```python
from build123d import *

# Parameters (mm, degrees)
ESBO_O1_W                = 50
ESBO_O1_H                = 11
RESSALTO_EXTRUS_O1_DEPTH = 22.5
ESBO_O2_W                = 46
ESBO_O2_H                = 7
CORTE_EXTRUS_O1_DEPTH    = 20.5
ESBO_O3_W                = 10.97916057
ESBO_O3_H                = 2
CORTE_EXTRUS_O2_DEPTH    = 4
CORTE_EXTRUS_O3_DEPTH    = 4
ESBO_O9_W                = 50
ESBO_O9_H                = 4
RESSALTO_EXTRUS_O4_DEPTH = 7
ESBO_O13_R               = 1.5
CORTE_EXTRUS_O4_DEPTH    = 7
ESBO_O19_W               = 9
ESBO_O19_H               = 4
RESSALTO_EXTRUS_O5_DEPTH = 22.5


with BuildPart() as part:
    # Esboço1 → Ressalto-extrusão1 (new body)
    with BuildSketch(Plane(origin=(0, 0, 0), x_dir=(1, 0, 0), z_dir=(0, 1, 0))):
        Rectangle(ESBO_O1_W, ESBO_O1_H)
    extrude(amount=RESSALTO_EXTRUS_O1_DEPTH)

    # Esboço2 → Corte-extrusão1 (cut)
    with BuildSketch(Plane(origin=(0, 22.5, 0), x_dir=(1, 0, 0), z_dir=(0, 1, 0))):
        Rectangle(ESBO_O2_W, ESBO_O2_H)
    extrude(amount=-CORTE_EXTRUS_O1_DEPTH, mode=Mode.SUBTRACT)

    # Esboço3 → Corte-extrusão2 (cut)
    with BuildSketch(Plane(origin=(0, 22.5, 0), x_dir=(1, 0, 0), z_dir=(0, 1, 0))):
        with Locations((0, 4.5)):
            Rectangle(ESBO_O3_W, ESBO_O3_H)
    extrude(amount=-CORTE_EXTRUS_O2_DEPTH, mode=Mode.SUBTRACT)

    # Esboço5 → Corte-extrusão3 (cut)
    with BuildSketch(Plane.XY.offset(5.5)):
        with BuildLine():
            Line((-21, 22.5), (-4.5, 22.5))
            Line((-4.5, 22.5), (-4.5, 11.75))
            ThreePointArc((-4.5, 11.75), (-12.75, 3.5), (-21, 11.75))
            Line((-21, 11.75), (-21, 22.5))
        make_face()
        with BuildLine():
            Line((4.5, 22.5), (21, 22.5))
            Line((21, 22.5), (21, 11.75))
            ThreePointArc((21, 11.75), (12.75, 3.5), (4.5, 11.75))
            Line((4.5, 11.75), (4.5, 22.5))
        make_face()
    extrude(amount=-CORTE_EXTRUS_O3_DEPTH, mode=Mode.SUBTRACT)

    # Esboço9 → Ressalto-extrusão4 (add)
    with BuildSketch(Plane(origin=(0, 0, -5.5), x_dir=(-1, 0, 0), z_dir=(0, 0, -1))):
        with Locations((0, 2)):
            Rectangle(ESBO_O9_W, ESBO_O9_H)
    extrude(amount=RESSALTO_EXTRUS_O4_DEPTH)

    # Esboço13 → Corte-extrusão4 (cut)
    with BuildSketch(Plane(origin=(0, 4, 0), x_dir=(1, 0, 0), z_dir=(0, 1, 0))):
        with Locations(Location((10, 9, 0), (0, 0, 270))):
            Circle(ESBO_O13_R)
        with Locations(Location((5, 9, 0), (0, 0, 270))):
            Circle(ESBO_O13_R)
        with Locations(Location((20, 9, 0), (0, 0, 270))):
            Circle(ESBO_O13_R)
        with Locations(Location((15, 9, 0), (0, 0, 270))):
            Circle(ESBO_O13_R)
        with Locations(Location((0, 9, 0), (0, 0, 270))):
            Circle(ESBO_O13_R)
        with Locations(Location((-5, 9, 0), (0, 0, 270))):
            Circle(ESBO_O13_R)
        with Locations(Location((-10, 9, 0), (0, 0, 270))):
            Circle(ESBO_O13_R)
        with Locations(Location((-15, 9, 0), (0, 0, 270))):
            Circle(ESBO_O13_R)
        with Locations(Location((-20, 9, 0), (0, 0, 270))):
            Circle(ESBO_O13_R)
    extrude(amount=-CORTE_EXTRUS_O4_DEPTH, mode=Mode.SUBTRACT)

    # Esboço19 → Ressalto-extrusão5 (add)
    with BuildSketch(Plane(origin=(0, 22.5, 0), x_dir=(1, 0, 0), z_dir=(0, 1, 0))):
        with Locations((0, -5.5)):
            Rectangle(ESBO_O19_W, ESBO_O19_H)
    extrude(amount=-RESSALTO_EXTRUS_O5_DEPTH)


solid = part.part
```
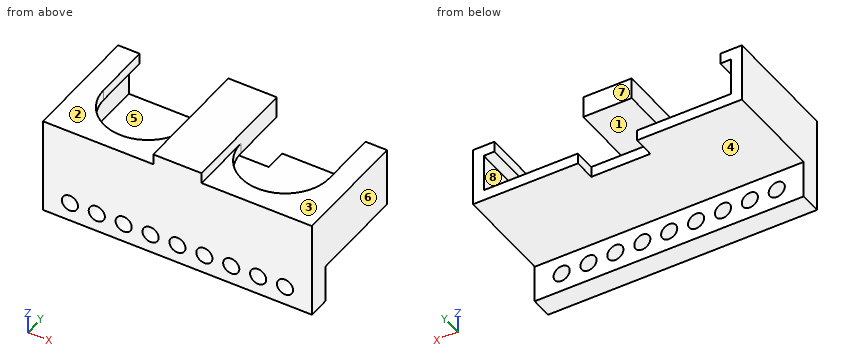
Design review of the part built by this model. Coordinates are the model's own, in mm. Face numbers are marked on the shaded views. A direction names the side the tool comes from. Give positions to 0.01 mm unless a question says otherwise; leave off trailing zeros. Loops run counter-clockwise (first coordinate to the right, second up) from the corner with the lowest first, then second, coordinate; pieces in that order, holes last. Notation, with made-up numbers: (58.25, 34) -> (104.25, 34) arc R19 ccw to (104.25, 48) -> close; hole circle Ø11 at (3, 63). An arc over 180 degrees is marked (long way). One line per item, written item: value.
Q1. Draft analysis for pull direction X (two halves, no side actions). For the marked faces 5, 6, 7 and 8, state which applies: pulls with the +X half, pulls with the -X half, needs draft (parallel to the pull), parting line crosses it, or undercut.
Numbers:
face 5: undercut
face 6: pulls with the +X half
face 7: needs draft
face 8: undercut
Q2. We need section D-D on z = -9. Give the number of separate pieces and of enclosed holes in the cut face, and give its area (3 significant figures).
Numbers:
separate pieces: 10
enclosed holes: 0
area: 92.0 mm^2
Q3. For pin 1 Ø2.5 at (x, z) = (10, -9) entering from +Y; pin 2 Ø2 at (x, y) = (-17.5, 13) entering from -Z; pin 3 Ø5 at (x, z) = (15, -9) entering from -Y; pin 4 Ø6 at (x, y) = (19, 15.5) entering from +Z, all flat-tipped, find the tip position at first contact; note any pin that passes through.
Numbers:
pin 1: passes through
pin 2: stops at z = -5.5
pin 3: stops at y = 0
pin 4: stops at z = 5.5
Q4. Machinability: for the marked faces 1, 2, 3 and 4, which of the approach directions +Z, -Z, +X, -X, +Y, -Y give a long, thin tool a straight path to every point of the face, cutting with its end or side? Answer none if there is none.
Numbers:
face 1: +Y
face 2: +Z, -X, +Y, -Y
face 3: +Z, +X, +Y, -Y
face 4: -Z, +X, -X, +Y
Q5. We need section C-C on x = -3. Give the boundary of the cut face in (y, z), and give its area (3 significant figures).
Numbers:
outline: (0, -12.5) -> (4, -12.5) -> (4, -5.5) -> (18.5, -5.5) -> (18.5, -3.5) -> (2, -3.5) -> (2, 3.5) -> (22.5, 3.5) -> (22.5, 7.5) -> (0, 7.5) -> close
area: 169 mm^2
Q6. We need section A-A on x = -15. Give the boundary of the cut face in (y, z).
Numbers:
outline: (0, -12.5) -> (4, -12.5) -> (4, -10.5) -> (0, -10.5) -> close; (0, -7.5) -> (4, -7.5) -> (4, -5.5) -> (22.5, -5.5) -> (22.5, -3.5) -> (2, -3.5) -> (2, 3.5) -> (3.81, 3.5) -> (3.81, 5.5) -> (0, 5.5) -> close
Q7. For L1, parallel to X at y = 14.25, z = -1.25; L2, parallel to X at y = 6, z = 4; L3, parallel to X at y = 11.5, z = 3.75, list the stretches that pass through material, from the lowest coordinate up.
Numbers:
L1: x = -25 to -23, 23 to 25
L2: x = -25 to -18.67, -6.83 to 6.83, 18.67 to 25
L3: x = -25 to -21, -4.5 to 4.5, 21 to 25
Q8. We need section B-B on y = 9. Give the boundary of the cut face in (x, z), and give its area (3 significant figures).
Numbers:
outline: (-25, -5.5) -> (25, -5.5) -> (25, 5.5) -> (20.53, 5.5) -> (20.53, 3.5) -> (23, 3.5) -> (23, -3.5) -> (-23, -3.5) -> (-23, 3.5) -> (-20.53, 3.5) -> (-20.53, 5.5) -> (-25, 5.5) -> close; (-4.97, 3.5) -> (4.97, 3.5) -> (4.97, 5.5) -> (4.5, 5.5) -> (4.5, 7.5) -> (-4.5, 7.5) -> (-4.5, 5.5) -> (-4.97, 5.5) -> close
area: 184 mm^2
